The model under review builds one solid part; all positions refer to its coordinate system, in mm. A direction names the side the tool comes from. Coordinates: 2 decimals unless noted, no trailing zeros. Write each loop counter-clockwise with the first axis right and the second up, starting at its lowest first coordinate (ties: lowest second). Pieces come first, ordered by that corner, then holes. Notation, with made-up numbers: (52.5, 30.25) - (106.5, 30.25) arc R20 ccw to (106.5, 35.25) - close; hole circle Ø7 at (-12.5, -4). An arc over 180 degrees is marked (long way). Return JSON: item names as keys, results as strings. Group by question number.
(1) We need section A-A on x = -0.55. Give the number of separate pieces and of enclosed holes in the cut face, then the cut area to 3 significant figures.
(2) To check wall thickness, follow L1, parallel to Z at x = -0.75, y = 0; L2, parallel to Z at x = 0.6, y = 0; L3, parallel to Z at x = -0.2, y = 0.2. State the ranges of each line that lie inside material, in increasing order. Write a range as from..to.
(3) For pin 1 Ø1.5 at (x, y) = (1, 1) entering from +Z, flat-tipped, find the tip position at first contact; note if it passes through.
(4) We need section B-B on z = 71. State the section outline as (x, y) points.
(5) Tool access review of faces 1 (the face through (0, 0, 97)), 2 (the face through (-0.194, 1.477, 49.554)): name each direction out of +Z, -Z, +X, -X, +Y, -Y from which nothing blocks a thin tool from reaching the whole face with its end or side.
```python
from build123d import *

# Parameters (mm, degrees)
SKETCH_1_R               = 1.49
EXTRUDE_1_DEPTH          = 100
CUT_EXTRUDE_3_DEPTH      = 101.022198536
CUT_EXTRUDE_3_DEPTH_BACK = 101.022198536
SKETCH_4_R               = 0.5
CUT_EXTRUDE_7_DEPTH      = 101.022198639
CUT_EXTRUDE_7_DEPTH_BACK = 101.022198639
SKETCH_2_W               = 1.49
SKETCH_2_H               = 6
SKETCH_6_R               = 0.5
CUT_EXTRUDE_8_DEPTH      = 10
SKETCH_7_R               = 1.49
CUT_EXTRUDE_9_DEPTH      = 0.5


with BuildPart() as part:
    # 草图1 → 凸台-拉伸1 (new body)
    with BuildSketch(Plane.XY):
        Circle(SKETCH_1_R)
    extrude(amount=EXTRUDE_1_DEPTH)

    # 草图4 → 切除-拉伸3 (cut, two sides: drawn at the far end of the back side and taken through both)
    with BuildSketch(Plane(origin=(0, 0, 0), x_dir=(0, 0, -1), z_dir=(1, 0, 0)).offset(-CUT_EXTRUDE_3_DEPTH_BACK)):
        with Locations((-2.5, 0)):
            Circle(SKETCH_4_R)
    extrude(amount=CUT_EXTRUDE_3_DEPTH + CUT_EXTRUDE_3_DEPTH_BACK, mode=Mode.SUBTRACT)

    # 草图2 → 切除-拉伸7 (cut, two sides: drawn at the far end of the back side and taken through both)
    with BuildSketch(Plane(origin=(0, 0, 0), x_dir=(1, 0, 0), z_dir=(0, 1, 0)).offset(-CUT_EXTRUDE_7_DEPTH_BACK)):
        with Locations((0.745, -97)):
            Rectangle(SKETCH_2_W, SKETCH_2_H)
    extrude(amount=CUT_EXTRUDE_7_DEPTH + CUT_EXTRUDE_7_DEPTH_BACK, mode=Mode.SUBTRACT)

    # 草图6 → 切除-拉伸8 (cut)
    with BuildSketch(Plane(origin=(0, 0, 0), x_dir=(0, 0, -1), z_dir=(1, 0, 0))):
        with BuildLine():
            Line((-100, 1.49), (-100, 0.01))
            ThreePointArc((-100, 0.01), (-99.566518036, 1.056518036), (-98.52, 1.49))
            Line((-98.52, 1.49), (-100, 1.49))
        make_face()
        with BuildLine():
            ThreePointArc((-98.52, -1.49), (-99.566518036, -1.056518036), (-100, -0.01))
            Line((-100, -0.01), (-100, -1.49))
            Line((-100, -1.49), (-98.52, -1.49))
        make_face()
        with Locations((-98.01, 0)):
            Circle(SKETCH_6_R)
    extrude(amount=-CUT_EXTRUDE_8_DEPTH, mode=Mode.SUBTRACT)

    # 草图7 → 切除-拉伸9 (cut)
    with BuildSketch(Plane(origin=(0, 0, 0), x_dir=(-1, 0, 0), z_dir=(0, 0, -1))):
        Circle(SKETCH_7_R)
    extrude(amount=-CUT_EXTRUDE_9_DEPTH, mode=Mode.SUBTRACT)


solid = part.part
```
Ans:
{
 "1": {"separate pieces": "1", "enclosed holes": "2", "area": "273 mm²"},
 "2": {"L1": "0.5..2, 3..97.51, 98.51..100", "L2": "0.5..2, 3..94", "L3": "0.5..2.04, 2.96..97.55, 98.47..99.99"},
 "3": {"pin 1": "z = 94"},
 "4": {"outline": "circle Ø2.98 at (0, 0)"},
 "5": {"face 1": "+Z, +X, +Y, -Y", "face 2": "+Z, -Z"}
}
